Can you work these out from the drawing? Everything is in mm from the part's minimum corner. Round coordinates to 2 decimals unless told otherwise and drop trailing zeros. Order: outer loops, then holes, each group sorted by start corner. A loop starts at its lowest first (then second) coordinate and runs counter-clockwise, first axis right, second up. Notation, with made-up numbers: M -7.75,82.5 L 48.25,82.5 A27 cw 48.25,115.5 Z; hole C -22.5,-8 d7. An arc over 180 degrees is marked long. Write each question's results on one line, items separated by ' | '. Start each with the question number.
1. Suppose I cut it at A-A on x = 28. Write out the boundary of the cut face in (y, z).
2. We'd pull the mould along Y, two halves only. Please class the marked faces 1, 2 and 3: released by +Y, released by -Y, zero draft, split by the parting line, or undercut.
3. Suppose I cut it at D-D on x = 153. Write out the boundary of the cut face in (y, z), and give its area (3 significant figures).
4. Please list where these lines run through material, in increasing order: L1, parallel to X at y = 16, z = 22.5 (1 decimal); L2, parallel to X at y = 18, z = 21 (1 decimal); L3, parallel to Y at x = 25, z = 18.5 (1 decimal).
5. Suppose I cut it at C-C on z = 4. Give the number of separate pieces and of enclosed holes in the cut face, and give its area (3 significant figures).
6. Suppose I cut it at B-B on y = 19.5. Write out the boundary of the cut face in (x, z) (1 decimal), and give its area (3 significant figures).
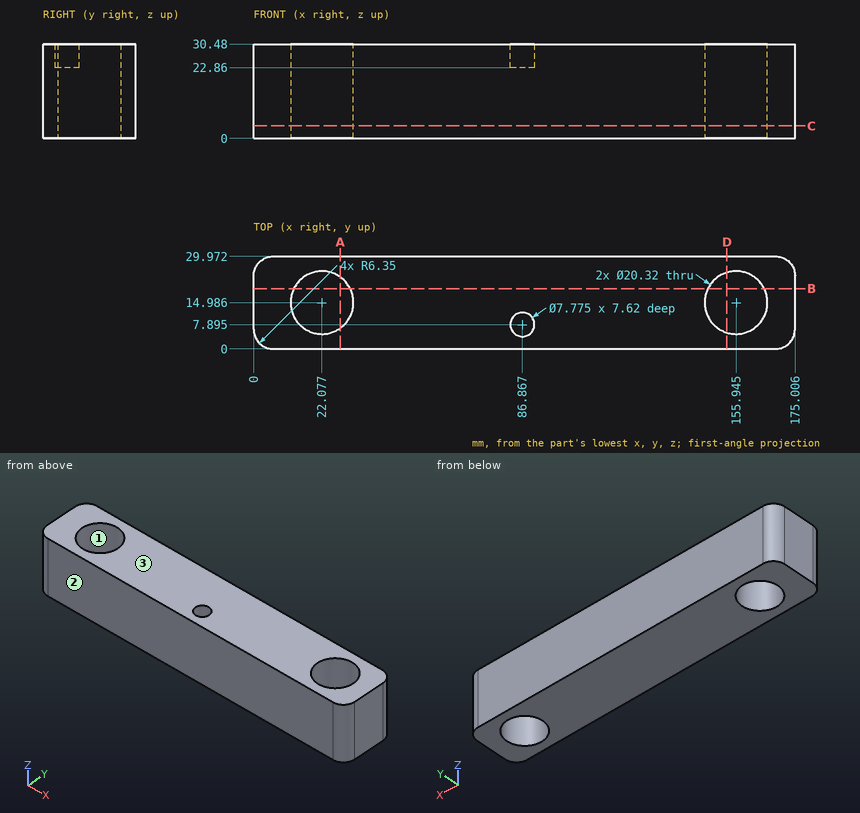
Filled sheet:
1) outline: M 0,0 L 6.73,0 L 6.73,30.48 L 0,30.48 Z; M 23.24,0 L 29.97,0 L 29.97,30.48 L 23.24,30.48 Z
2) face 1: undercut | face 2: released by -Y | face 3: zero draft
3) outline: M 0,0 L 5.26,0 L 5.26,30.48 L 0,30.48 Z; M 24.71,0 L 29.97,0 L 29.97,30.48 L 24.71,30.48 Z | area: 321 mm^2
4) L1: x = 0 to 12, 32.2 to 145.8, 166.1 to 175 | L2: x = 0 to 12.4, 31.8 to 146.2, 165.6 to 175 | L3: y = 0 to 5.3, 24.7 to 30
5) separate pieces: 1 | enclosed holes: 2 | area: 4,560 mm^2
6) outline: M 0,0 L 13,0 L 13,30.5 L 0,30.5 Z; M 31.2,0 L 146.8,0 L 146.8,30.5 L 31.2,30.5 Z; M 165,0 L 175,0 L 175,30.5 L 165,30.5 Z | area: 4,220 mm^2
